```python
from build123d import *

# Parameters (mm, degrees)
SKETCH1_W           = 20
SKETCH1_H           = 300
SKETCH1_R           = 5
BOSS_EXTRUDE2_DEPTH = 10
SKETCH5_W           = 40
SKETCH5_H           = 40
BOSS_EXTRUDE3_DEPTH = 10


with BuildPart() as part:
    # Sketch1 → Boss-Extrude2 (new, symmetric)
    with BuildSketch(Plane.XY):
        with Locations((10, 150)):
            Rectangle(SKETCH1_W, SKETCH1_H)
        with Locations((10, 290)):
            Circle(SKETCH1_R, mode=Mode.SUBTRACT)
    extrude(amount=BOSS_EXTRUDE2_DEPTH, both=True)

    # Sketch5 → Boss-Extrude3 (add, symmetric)
    with BuildSketch(Plane(origin=(0, 0, 0), x_dir=(1, 0, 0), z_dir=(0, 1, 0))):
        with Locations((10, 0)):
            Rectangle(SKETCH5_W, SKETCH5_H)
    extrude(amount=BOSS_EXTRUDE3_DEPTH, both=True)


solid = part.part
```
The listing builds one solid part. Answer for the finished solid, in the listing's coordinates (mm). A direction names the side the tool comes from. Round coordinates to 2 decimals unless told otherwise and drop trailing zeros. Write each loop counter-clockwise with the first axis right and the second up, starting at its lowest first coordinate (ties: lowest second). Pieces come first, ordered by that corner, then holes. Notation, with made-up numbers: (-38, 5) -> (-24, 5) arc R14 cw to (-24, 14) -> close; hole circle Ø5 at (-23, 58.25). An arc over 180 degrees is marked (long way). Answer as a JSON object with one key per item and string values. Group by question number.
Q1. Section D-D (y = 251.5) is taken. Write down the section's boundary in (x, z).
Q2. Straight lines are drawn through the part: line 1 along Y through (x, z) = (10, 2.75); line 2 along X through (y, z) = (290, 2.25); line 3 along Z through (x, y) = (12, 135). For each, find the intervals that lie inside material, in ascending order.
Q3. Each of these flat-tipped pins is pushed along its axis until it touches: pin 1 Ø10 at (x, y) = (6.5, 88) entering from -Z; pin 2 Ø12 at (y, z) = (168.5, -15.5) entering from -X; pin 3 Ø16 at (y, z) = (227, 3.5) entering from +X. Where does it stop, or does it pass through?
Q4. Determine the mould class of faces 5 (the face through (20, 153, 0)), 6 (the face through (10, 10, -14)), 7 (the face through (9.349, 294.957, -0.14)) for opening direction X: pulls with the +X half, pulls with the -X half, needs draft (parallel to the pull), parting line crosses it, or undercut.
Q5. Which of the six approach directions +Z, -Z, +X, -X, +Y, -Y give full straight-line access (tool end or side, diameter ignored) to faces 1 (the face through (0, 153, 0)), 2 (the face through (10, 157, 10)), 3 (the face through (10, 0, 20)), 4 (the face through (10, 157, -10))?
Q6. Section B-B (y = 290) is taken. Write down the section's boundary in (x, z), plus the area to 3 significant figures.
Q7. Section A-A (x = 10) is taken. Write down the section's boundary in (y, z), plus the area to 3 significant figures.
Q8. Section C-C (z = -3) is taken. Write down the section's boundary in (x, y).
Check values:
{
 "1": {"outline": "(0, -10) -> (20, -10) -> (20, 10) -> (0, 10) -> close"},
 "2": {"line 1": "-10 to 285, 295 to 300", "line 2": "0 to 5, 15 to 20", "line 3": "-10 to 10"},
 "3": {"pin 1": "z = -10", "pin 2": "x = 0", "pin 3": "x = 20"},
 "4": {"face 5": "pulls with the +X half", "face 6": "needs draft", "face 7": "undercut"},
 "5": {"face 1": "+Z, -Z, -X, +Y", "face 2": "+Z, +X, -X, +Y", "face 3": "+Z, +X, -X, +Y, -Y", "face 4": "-Z, +X, -X, +Y"},
 "6": {"outline": "(0, -10) -> (5, -10) -> (5, 10) -> (0, 10) -> close; (15, -10) -> (20, -10) -> (20, 10) -> (15, 10) -> close", "area": "200 mm^2"},
 "7": {"outline": "(-10, -20) -> (10, -20) -> (10, -10) -> (285, -10) -> (285, 10) -> (10, 10) -> (10, 20) -> (-10, 20) -> close; (295, -10) -> (300, -10) -> (300, 10) -> (295, 10) -> close", "area": "6,400 mm^2"},
 "8": {"outline": "(-10, -10) -> (30, -10) -> (30, 10) -> (20, 10) -> (20, 300) -> (0, 300) -> (0, 10) -> (-10, 10) -> close; hole circle Ø10 at (10, 290)"}
}
